Design review of the part built by this model. Coordinates are the model's own, in mm. Face numbers are marked on the shaded views. A direction names the side the tool comes from. Round coordinates to 2 decimals unless told otherwise and drop trailing zeros. Loops run counter-clockwise (first coordinate to the right, second up) from the corner with the lowest first, then second, coordinate; pieces in that order, holes last. Notation, with made-up numbers: (-38.75, 86.5) -> (-14.75, 86.5) arc R17 ccw to (-14.75, 90.5) -> close; hole circle Ø11 at (84.25, 57.25). An arc over 180 degrees is marked (long way). Answer as CSV lines item,"result". Start each with the question number.
(1) Take a section at A-A, the plane x = 36. Write out the cut boundary in (y, z) (3 decimals), and give its area (3 significant figures).
(2) Draft analysis for pull direction Z (two halves, no side actions). For the marked faces 1, 2, 3 and 4, state which applies: +Z half, -Z half, draft (parallel to the pull), parting line (faces both ways), or undercut.
(3) For P1, Ø6, axis at y = 5.5, z = 15, coming from the -X side; P2, Ø2, axis at x = -100, z = 17, coming from the -Y side; P3, Ø8, axis at y = 28.5, z = -1, coming from the -X side; P4, Ø4, axis at y = 32.5, z = -7.5, coming from the +X side (3 decimals), all flat-tipped, find the tip position at first contact; note any pin that passes through.
(4) Take a section at C-C, the plane z = 14. Write out the cut boundary in (x, y).
(5) To check wall thickness, follow line 1 (X direction, y = 0, z = -4); line 2 (Z direction, x = -108, y = -25) (3 decimals); line 3 (X direction, y = 0, z = -11). State the ranges of each line that lie inside material, in increasing order. Write a range as from..to.
(6) Machinability: for the marked faces 5 and 6, which of the approach directions +Z, -Z, +X, -X, +Y, -Y give a long, thin tool a straight path to every point of the face, cutting with its end or side? Answer none if there is none.
(7) Take a section at D-D, the plane y = 28.5. Write out the cut boundary in (x, z) (3 decimals), and give its area (3 significant figures).
(8) Take a section at B-B, the plane y = -25.4. Write out the cut boundary in (x, z) (3 decimals).
Autodesk Inventor part; units mm, degrees
ref_plane "YZ Plane" through (0, 0, 0) normal (1, 0, 0) x (0, 1, 0)
ref_plane "XZ Plane" through (0, 0, 0) normal (0, 1, 0) x (-1, 0, 0)
ref_plane "XY Plane" through (0, 0, 0) normal (0, 0, 1) x (1, 0, 0)
sketch "Sketch1" plane through (0, 0, 0) normal (0, 0, 1) x (1, 0, 0)
  circle A0 centre (0, 0) radius 50.8
  line L0 (0, -50.8) -> (-127, -50.8)
  line L1 (-127, -50.8) -> (-127, 0)
  line L2 (-127, 0) -> (-20.32, 46.559)
  dimension "d0" = 127
  dimension "d1" = 101.6
  dimension "d2" = 50.8
extrude "MAIN BODY" add sketch "Sketch1" along normal mid plane 19.05
sketch "Sketch2" plane through (0, 0, 0) normal (0, 0, 1) x (1, 0, 0)
  arc A0 (0, -50.8) -> (-20.32, 46.559) centre (0, 0) ccw
  circle A1 centre (0, 0) radius 50.8
  point P0 (0, -50.8)
  dimension "d5" = 101.6
extrude "MAIN BODY LIP" add sketch "Sketch2" along normal mid plane 38.1
sketch "Sketch3" plane through (0, 0, 9.525) normal (0, 0, 1) x (1, 0, 0)
  line L0 (-127, -50.8) -> (0, -50.8)
  line L1 (-127, -50.8) -> (-101.6, -50.8)
  line L2 (-101.6, -50.8) -> (-101.6, 0)
  line L3 (-101.6, 0) -> (-127, 0)
  line L4 (-127, 0) -> (-127, -50.8)
  point P0 (0, 0)
  point P1 (-101.6, -25.4)
  dimension "d8" = 25.4
  dimension "d9" = 50.8
extrude "SIDE EXT" add sketch "Sketch3" along normal blind 31.75
sketch "Sketch4" plane through (-101.6, -50.8, 9.525) normal (1, 0, 0) x (0, 0, -1)
  line L0 (-31.75, 0) -> (-31.75, 50.8)
  circle A0 centre (-31.75, 25.4) radius 25.4
  point P0 (9.525, 50.8)
extrude "SIDE EXT CURVE" add sketch "Sketch4" against normal blind 25.4 contours A0 L0 picked at (-40.1549, 26.4205)
sketch "Sketch5" plane through (-101.6, -50.8, 9.525) normal (1, 0, 0) x (0, 0, -1)
  arc A0 (-31.75, 50.8) -> (-31.75, 0) centre (-31.75, 25.4) ccw
  point P0 (9.525, 50.8)
hole "SIDE EXT HOLE" at (-101.6, -25.4, 41.275) direction (-1, 0, 0) diameter 25.4 end through all
sketch "Sketch6" plane through (0, 0, 19.05) normal (0, 0, 1) x (1, 0, 0)
  circle A0 centre (0, 0) radius 50.8
hole "MAIN BODY HOLE" at (0, 0, 19.05) direction (0, 0, -1) diameter 76.2 end through all
properties part number "ANS7-4-BK" material "PET Plastic"
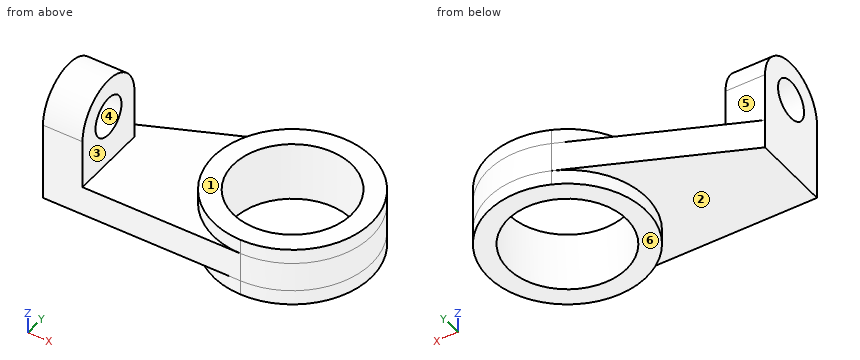
The answers:
1,outline,"(-35.842, -19.05) -> (-12.474, -19.05) -> (-12.474, 19.05) -> (-35.842, 19.05) -> (-35.842, 9.525) -> close; (12.474, -19.05) -> (35.842, -19.05) -> (35.842, 9.525) -> (35.842, 19.05) -> (12.474, 19.05) -> close"
1,area,"1,780 mm²"
2,face 1,"+Z half"
2,face 2,"-Z half"
2,face 3,"draft"
2,face 4,"undercut"
3,P1,"x = -50.74"
3,P2,"through"
3,P3,"x = -70.86"
3,P4,"x = 40.625"
4,outline,"(-127, -50.8) -> (-101.6, -50.8) -> (-101.6, 0) -> (-127, 0) -> close; (-20.32, 46.56) arc R50.8 ccw to (0, -50.8) arc R50.8 ccw (long way) to start; hole circle Ø76.2 at (0, 0)"
5,line 1,"-127..-38.1, 38.1..50.8"
5,line 2,"-9.525..28.581, 53.969..66.672"
5,line 3,"-50.8..-38.1, 38.1..50.8"
6,face 5,"+Z, -X, +Y"
6,face 6,"-Z, +X, -X, +Y, -Y"
7,outline,"(-61.698, -9.525) -> (-42.052, -9.525) -> (-42.052, -19.05) -> (-25.286, -19.05) -> (-25.286, 19.05) -> (-42.052, 19.05) -> (-42.052, 9.525) -> (-61.698, 9.525) -> close; (25.286, -19.05) -> (42.052, -19.05) -> (42.052, 9.525) -> (42.052, 19.05) -> (25.286, 19.05) -> close"
7,area,"1,650 mm²"
8,outline,"(-127, -9.525) -> (-43.994, -9.525) -> (-43.994, -19.05) -> (-28.398, -19.05) -> (-28.398, 19.05) -> (-43.994, 19.05) -> (-43.994, 9.525) -> (-101.6, 9.525) -> (-101.6, 28.575) -> (-127, 28.575) -> close; (-127, 53.975) -> (-101.6, 53.975) -> (-101.6, 66.675) -> (-127, 66.675) -> close; (28.398, -19.05) -> (43.994, -19.05) -> (43.994, 9.525) -> (43.994, 19.05) -> (28.398, 19.05) -> close"
